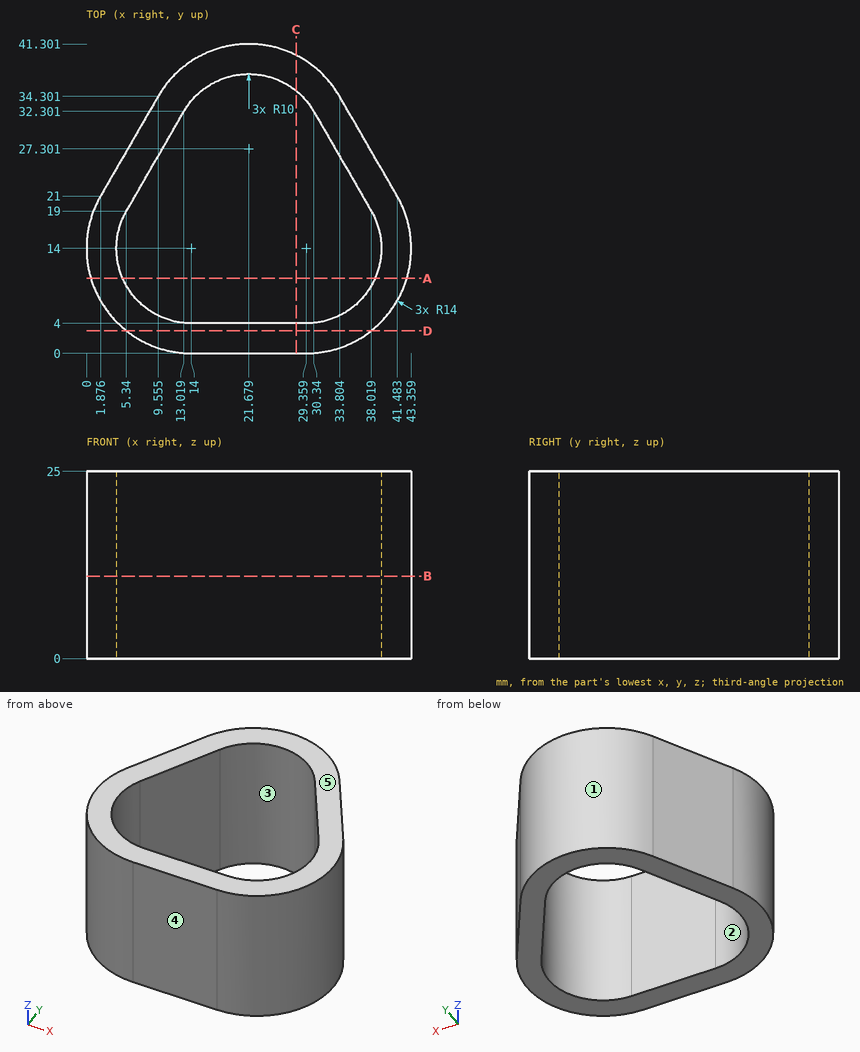
Job drawing, mm, ordinate dimensions from the low corner. One solid piece. A direction names the side the tool comes from. Round coordinates to 2 decimals unless told otherwise and drop trailing zeros. Loops run counter-clockwise (first coordinate to the right, second up) from the corner with the lowest first, then second, coordinate; pieces in that order, holes last.
Item 1: Mould opens along Y. For the marked faces 3, 4 and 5 say: +Y half, -Y half, draft (parallel to the pull), parting line (faces both ways), or undercut.
Item 2: Cut at A-A, the plane y = 10. Give the cut face in (x, z) (1 decimal).
Item 3: Cut at D-D, the plane y = 3. Give the cut face in (x, z).
Item 4: 3-axis set-ups, long thin cutter, end or side, ignore diameter. For the marked faces 1 and 2: which of +Z, -Z, +X, -X, +Y, -Y reach the whole face in a straight line?
Item 5: Drop flat-ended pins along their axis: P1, Ø4, axis at y = 8.5, z = 19, coming from the +X side (1 decimal); P2, Ø5, axis at y = 30, z = 19, coming from the -X side; P3, Ø2, axis at y = 23, z = 3.5, coming from the +X side (1 decimal). Give the stop position or say it passes through.
Item 6: Drill centre lines: line 1 (Y direction, x = 9, z = 5.75) (1 decimal); line 2 (Y direction, x = 12, z = 4.25) (1 decimal); line 3 (X direction, y = 7.5, z = 15). Where is each one in solid material? Low to high.
Item 7: Cut at B-B, the plane z = 11. Give the cut face in (x, y) (1 decimal), then the cut area to 3 significant figures.
Item 8: Cut at C-C, the plane x = 28. Give the cut face in (y, z).
A:
1. face 3: undercut
1. face 4: -Y half
1. face 5: draft
2. outline: (0.6, 0) - (4.8, 0) - (4.8, 25) - (0.6, 25) - close; (38.5, 0) - (42.8, 0) - (42.8, 25) - (38.5, 25) - close
3. outline: (5.34, 0) - (38.02, 0) - (38.02, 25) - (5.34, 25) - close
4. face 1: +Z, -Z, +Y
4. face 2: +Z, -Z
5. P1: stops at x = 42.9
5. P2: stops at x = 5.63
5. P3: stops at x = 40.9
6. line 1: y = 0.9 to 5.3, 25.3 to 33.3
6. line 2: y = 0.1 to 4.2, 30.5 to 37.4
6. line 3: x = 1.6 to 6.4, 36.96 to 41.76
7. outline: (1.9, 21) arc R14 ccw to (14, 0) - (29.4, 0) arc R14 ccw to (41.5, 21) - (33.8, 34.3) arc R14 ccw to (9.6, 34.3) - close; hole (5.3, 19) arc R10 ccw to (14, 4) - (29.4, 4) arc R10 ccw to (38, 19) - (30.3, 32.3) arc R10 ccw to (13, 32.3) - close
7. area: 486 mm2
8. outline: (0, 0) - (4, 0) - (4, 25) - (0, 25) - close; (35.05, 0) - (39.79, 0) - (39.79, 25) - (35.05, 25) - close
